Could you check a few things on this model? Use its own coordinates, in mm. A direction names the side the tool comes from. Give positions to 0.01 mm unless a question says otherwise; leave off trailing zeros. Write each loop counter-clockwise with the first axis right and the second up, starting at its lowest first coordinate (ties: lowest second). Pieces come first, ordered by that corner, then holes. Notation, with made-up numbers: (76, 70) - (117, 70) arc R23 ccw to (117, 85) - close; hole circle Ø4 at (48.25, 78.25). An arc over 180 degrees is marked (long way). Answer as CSV lines item,"result". Start each with the question number.
Q1. If I drill on line 1 along Z through (x, y) = (54, 57); line 2 along X through (y, z) = (52, 21); line 3 along Y through (x, z) = (-98, 82.5), over which ranges is the centre line in solid material (lowest first)?
Q2. Imagine slicing it at C-C on x = -154.5. List the corners of the cut face in (y, z) for me.
Q3. Imagine slicing it at A-A on y = 35. List the corners of the cut face in (x, z) for me.
Q4. Imagine slicing it at B-B on z = 89.5. List the corners of the cut face in (x, y) for me.
Q5. Will these pins go through, and if not, where does the flat tip stop? pin 1 Ø1 at (x, z) = (-128, 0) entering from +Y; pin 2 Ø4 at (y, z) = (16.5, 104) entering from -X.
Q6. We'd pull the mould along Z, two halves only. Please class faces 1 (the face through (-224.8, 49.7, -142.7)), 2 (the face through (-3, 0, -2)), 3 (the face through (-3, 25, -135)), 4 (the face through (219.06, 20.52, 138.96)): pulls with the +Z half, pulls with the -Z half, needs draft (parallel to the pull), parting line crosses it, or undercut.
Q7. On a 3-axis mill with a long thin cutter (end or side, diameter ignored), from which of +Z, -Z, +X, -X, +Y, -Y can I reach the whole of each face in a straight line? I mean faces 5 (the face through (240, 50, 2)), 6 (the face through (-215, 55, 135)). Say none if no direction works.
```python
from build123d import *

# Parameters (mm, degrees)
SKETCH1_W           = 480
SKETCH1_H           = 315
BOSS_EXTRUDE1_DEPTH = 70
SKETCH3_W           = 460
SKETCH3_H           = 300
CUT_EXTRUDE1_DEPTH  = 60
CHAMFER1_SIZE       = 30


with BuildPart() as part:
    # Sketch1 → Boss-Extrude1 (new body)
    with BuildSketch(Plane(origin=(0, 0, 0), x_dir=(1, 0, 0), z_dir=(0, 1, 0))):
        Rectangle(SKETCH1_W, SKETCH1_H)
    extrude(amount=BOSS_EXTRUDE1_DEPTH)

    # Sketch3 → Cut-Extrude1 (cut)
    with BuildSketch(Plane(origin=(0, 70, 0), x_dir=(1, 0, 0), z_dir=(0, 1, 0))):
        Rectangle(SKETCH3_W, SKETCH3_H)
    extrude(amount=-CUT_EXTRUDE1_DEPTH, mode=Mode.SUBTRACT)

    # Chamfer1
    chamfer1_edges = [part.edges().sort_by_distance(p)[0] for p in [
        (230, 10, 0),
        (230, 40, -150),
        (0, 10, 150),
        (230, 40, 150),
        (-230, 10, 0),
        (-230, 40, 150),
        (0, 10, -150),
        (-230, 40, -150),
        (0, 0, -157.5),
        (240, 0, 0),
        (0, 0, 157.5),
        (-240, 0, 0),
        (-240, 35, -157.5),
        (240, 35, -157.5),
        (240, 35, 157.5),
        (-240, 35, 157.5),
    ]]
    chamfer(chamfer1_edges, length=CHAMFER1_SIZE)


solid = part.part
```
Conclusion:
1,line 1,"-157.5 to -150, 150 to 157.5"
1,line 2,"-240 to -230, 230 to 240"
1,line 3,"0 to 10"
2,outline,"(0, -127.5) - (30, -157.5) - (70, -157.5) - (70, -150) - (40, -150) - (10, -120) - (10, 120) - (40, 150) - (70, 150) - (70, 157.5) - (30, 157.5) - (0, 127.5) - close"
3,outline,"(-240, -127.5) - (-210, -157.5) - (210, -157.5) - (240, -127.5) - (240, 127.5) - (210, 157.5) - (-210, 157.5) - (-240, 127.5) - close; hole (-225, -120) - (-200, -145) - (200, -145) - (225, -120) - (225, 120) - (200, 145) - (-200, 145) - (-225, 120) - close"
4,outline,"(-240, 30) - (-210, 0) - (210, 0) - (240, 30) - (240, 70) - (230, 70) - (230, 40) - (200, 10) - (-200, 10) - (-230, 40) - (-230, 70) - (-240, 70) - close"
5,pin 1,"y = 10"
5,pin 2,"x = -228.5"
6,face 1,"pulls with the -Z half"
6,face 2,"needs draft"
6,face 3,"undercut"
6,face 4,"pulls with the +Z half"
7,face 5,"+Z, -Z, +X, +Y, -Y"
7,face 6,"+Y"
